Autodesk Inventor part; units mm, degrees
ref_plane "YZ Plane" through (0, 0, 0) normal (1, 0, 0) x (0, 1, 0)
ref_plane "XZ Plane" through (0, 0, 0) normal (0, 1, 0) x (-1, 0, 0)
ref_plane "XY Plane" through (0, 0, 0) normal (0, 0, 1) x (1, 0, 0)
sketch "Sketch1" plane through (0, 0, 0) normal (1, 0, 0) x (0, 1, 0)
  line L0 (10.4423, 8.7344) -> (-40.3577, 8.7344)
  line L1 (-40.3577, 8.7344) -> (-40.3577, -16.6656)
  line L2 (-40.3577, -16.6656) -> (10.4423, -16.6656)
  line L3 (10.4423, -16.6656) -> (10.4423, 8.7344)
  line L4 (7.3181, 5.6102) -> (-37.2335, 5.6102)
  line L5 (-37.2335, 5.6102) -> (-37.2335, -13.5414)
  line L6 (-37.2335, -13.5414) -> (7.3181, -13.5414)
  line L7 (7.3181, -13.5414) -> (7.3181, 5.6102)
  point P0 (0, 0)
  dimension "d0" = 50.8
  dimension "d1" = 25.4
  dimension "d2" = 3.1242
extrude "Extrusion1" add sketch "Sketch1" along normal blind 711.2
sketch "Sketch2" plane through (0, 10.4423, 8.7344) normal (0, 1, 0) x (1, 0, 0)
  line L0 (0, 25.4) -> (22.2758, 3.1242)
  line L1 (0, 3.1242) -> (711.2, 3.1242)
  line L2 (0, 25.4) -> (31.5027, 25.4) construction
  line L3 (22.2758, 3.1242) -> (38.5716, -13.1716)
  line L4 (0, 0) -> (711.2, 0)
  line L5 (25.4, 0) -> (0, 0)
  line L6 (0, 0) -> (0, 25.4)
  line L7 (711.2, 25.4) -> (678.2071, -7.5929)
  line L8 (711.2, 25.4) -> (757.859, 25.4) construction
  line L9 (685.8, 0) -> (711.2, 0)
  line L10 (711.2, 0) -> (711.2, 25.4)
  line L11 (711.2, 25.4) -> (711.2, 0)
  point P0 (0, 8.7344)
  dimension "d5" = 45
  dimension "d6" = 135
extrude "Extrusion2" cut sketch "Sketch2" against normal blind 711.2 contours L0 L1 L6 | L3 L4 L6 L1
extrude "Extrusion3" cut sketch "Sketch2" against normal blind 711.2 contours L7 L10 L1 | L1 L10 L4 L7
properties part number "28in 1x2"
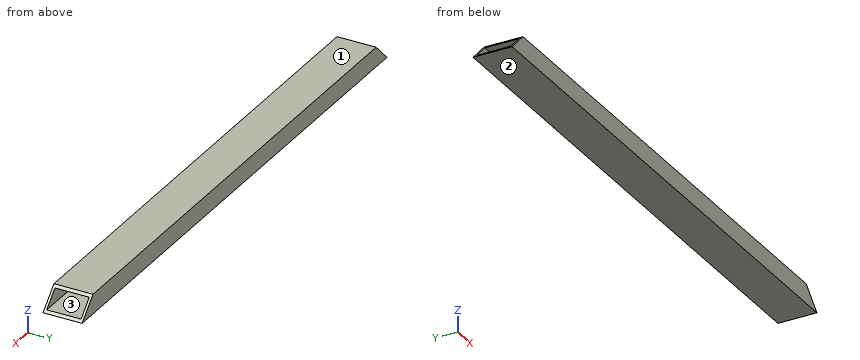
Source: CAD feature listing. Evaluate the final solid. Frame: model axes, mm. Face numbers are marked on the shaded views. Round coordinates to 2 decimals unless told otherwise and drop trailing zeros. Loops run counter-clockwise (first coordinate to the right, second up) from the corner with the lowest first, then second, coordinate; pieces in that order, holes last.
Q1. Ray query, line 1 (Z direction, x = 636.5, y = -3); line 2 (Y direction, x = 341.5, z = -1.5); line 3 (X direction, y = -32, z = 7). Return the intervals inside material, ascending.
Q2. Section C-C, the plane x = 353. Return loops of the section in (y, z).
Q3. Mould query, pull axis Z, two halves, no side actions, for the marked faces 1, 2 and 3. Classes: pulls with the +Z half, pulls with the -Z half, needs draft (parallel to the pull), parting line crosses it, or undercut.
Q4. Section B-B, the plane z = -7. Return loops of the section in (x, y).
Q5. Section A-A, the plane y = -8.5. Return loops of the section in (x, z), plus the area to 3 significant figures.
Solutions:
1. line 1: z = -16.67 to -13.54, 5.61 to 8.73
1. line 2: y = -40.36 to -37.23, 7.32 to 10.44
1. line 3: x = 23.67 to 687.53
2. outline: (-40.36, -16.67) - (10.44, -16.67) - (10.44, 8.73) - (-40.36, 8.73) - close; hole (-37.23, -13.54) - (7.32, -13.54) - (7.32, 5.61) - (-37.23, 5.61) - close
3. face 1: pulls with the +Z half
3. face 2: pulls with the -Z half
3. face 3: undercut
4. outline: (9.67, -40.36) - (701.53, -40.36) - (701.53, -37.23) - (9.67, -37.23) - close; (9.67, 7.32) - (701.53, 7.32) - (701.53, 10.44) - (9.67, 10.44) - close
5. outline: (0, -16.67) - (711.2, -16.67) - (708.08, -13.54) - (3.12, -13.54) - close; (22.28, 5.61) - (688.92, 5.61) - (685.8, 8.73) - (25.4, 8.73) - close
5. area: 4,290 mm2
